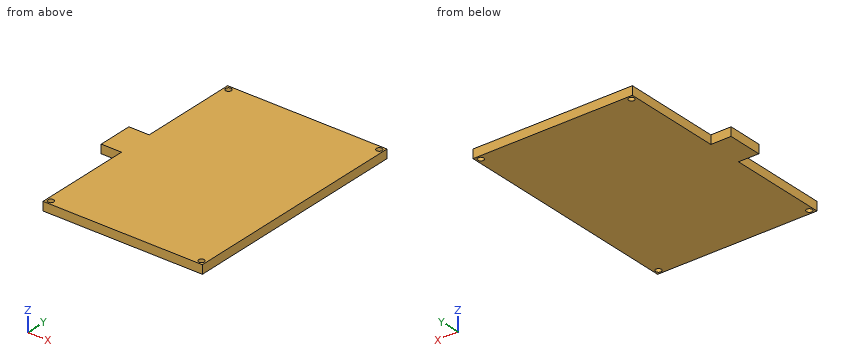
```python
from build123d import *

# Parameters (mm, degrees)
BOSS_EXTRUDE1_DEPTH = 3
SKETCH2_R           = 1
CUT_EXTRUDE1_DEPTH  = 56


with BuildPart() as part:
    # Sketch1 → Boss-Extrude1 (new body)
    with BuildSketch(Plane.XY):
        Polygon((-34.5, -6), (-27.5, -6), (-27.5, -40), (27.5, -40), (27.5, 40), (-27.5, 40), (-27.5, 6), (-34.5, 6), align=None)
    extrude(amount=-BOSS_EXTRUDE1_DEPTH)

    # Sketch2 → Cut-Extrude1 (cut)
    with BuildSketch(Plane.XY):
        with Locations((-26, -38.5)):
            Circle(SKETCH2_R)
        with Locations((26, -38.5)):
            Circle(SKETCH2_R)
        with Locations((26, 38.5)):
            Circle(SKETCH2_R)
        with Locations((-26, 38.5)):
            Circle(SKETCH2_R)
    extrude(amount=-CUT_EXTRUDE1_DEPTH, mode=Mode.SUBTRACT)


solid = part.part
```
The model under review builds one solid part; all positions refer to its coordinate system, in mm. Coordinates: 2 decimals unless noted, no trailing zeros. Write each loop counter-clockwise with the first axis right and the second up, starting at its lowest first coordinate (ties: lowest second). Pieces come first, ordered by that corner, then holes.
1) Clearance check with flat-ended pins moving along their axes: pin 1 Ø0.9 at (y, z) = (-16, -1) entering from -X; pin 2 Ø1.5 at (x, z) = (-30.5, -1) entering from -Y. State where each tip first meets the part, or that it passes through.
2) To check wall thickness, follow probe 1 along Y at (x, z) = (-26, -2); probe 2 along X at (y, z) = (35.5, -1.4). State the ranges of each line that lie inside material, in increasing order.
3) We need section B-B on z = -1.7. State the section outline as (x, y) points, then the cut area to 3 significant figures.
4) We need section A-A on x = -26. State the section outline as (y, z) points.
5) We need section C-C on y = -38.5. State the section outline as (x, z) points.
Answer list:
1. pin 1: stops at x = -27.5
1. pin 2: stops at y = -6
2. probe 1: y = -40 to -39.5, -37.5 to 37.5, 39.5 to 40
2. probe 2: x = -27.5 to 27.5
3. outline: (-34.5, -6) - (-27.5, -6) - (-27.5, -40) - (27.5, -40) - (27.5, 40) - (-27.5, 40) - (-27.5, 6) - (-34.5, 6) - close; hole circle Ø2 at (-26, -38.5); hole circle Ø2 at (-26, 38.5); hole circle Ø2 at (26, -38.5); hole circle Ø2 at (26, 38.5)
3. area: 4,470 mm2
4. outline: (-40, -3) - (-39.5, -3) - (-39.5, 0) - (-40, 0) - close; (-37.5, -3) - (37.5, -3) - (37.5, 0) - (-37.5, 0) - close; (39.5, -3) - (40, -3) - (40, 0) - (39.5, 0) - close
5. outline: (-27.5, -3) - (-27, -3) - (-27, 0) - (-27.5, 0) - close; (-25, -3) - (25, -3) - (25, 0) - (-25, 0) - close; (27, -3) - (27.5, -3) - (27.5, 0) - (27, 0) - close
